Check sheet for the modelled part. Datum: model origin and axes. Units: mm. Coordinates: 2 decimals unless noted, no trailing zeros. Loops run counter-clockwise (first coordinate to the right, second up) from the corner with the lowest first, then second, coordinate; pieces in that order, holes last. Notation, with made-up numbers: (22, -39.75) -> (29, -39.75) arc R23 cw to (29, -5.75) -> close; hole circle Ø1 at (63.5, 17). An arc over 180 degrees is marked (long way). Use CSV: the item, a comma, the result in double quotes.
```python
from build123d import *

# Parameters (mm, degrees)
BOSS_EXTRUDE1_DEPTH = 60


with BuildPart() as part:
    # Sketch1 → Boss-Extrude1 (new body)
    with BuildSketch(Plane.XY.offset(12.5)):
        with BuildLine():
            Line((1.189339828, 2), (-1.189339828, 2))
            ThreePointArc((-1.189339828, 2), (-1.285010686, 2.019030117), (-1.366116524, 2.073223305))
            Line((-1.366116524, 2.073223305), (-3.116116524, 3.823223305))
            ThreePointArc((-3.116116524, 3.823223305), (-3.189339828, 4), (-3.116116524, 4.176776695))
            Line((-3.116116524, 4.176776695), (-2.292893219, 5))
            Line((-2.292893219, 5), (-3.094974747, 5))
            Line((-3.094974747, 5), (-3.623223305, 4.471751442))
            ThreePointArc((-3.623223305, 4.471751442), (-3.8, 4.398528137), (-3.976776695, 4.471751442))
            Line((-3.976776695, 4.471751442), (-4.505025253, 5))
            Line((-4.505025253, 5), (-4.75, 5))
            ThreePointArc((-4.75, 5), (-4.926776695, 4.926776695), (-5, 4.75))
            Line((-5, 4.75), (-5, 4.505025253))
            Line((-5, 4.505025253), (-4.471751442, 3.976776695))
            ThreePointArc((-4.471751442, 3.976776695), (-4.398528137, 3.8), (-4.471751442, 3.623223305))
            Line((-4.471751442, 3.623223305), (-5, 3.094974747))
            Line((-5, 3.094974747), (-5, 2.292893219))
            Line((-5, 2.292893219), (-4.176776695, 3.116116524))
            ThreePointArc((-4.176776695, 3.116116524), (-4, 3.189339828), (-3.823223305, 3.116116524))
            Line((-3.823223305, 3.116116524), (-2.073223305, 1.366116524))
            ThreePointArc((-2.073223305, 1.366116524), (-2.019030117, 1.285010686), (-2, 1.189339828))
            Line((-2, 1.189339828), (-2, -1.189339828))
            ThreePointArc((-2, -1.189339828), (-2.019030117, -1.285010686), (-2.073223305, -1.366116524))
            Line((-2.073223305, -1.366116524), (-3.823223305, -3.116116524))
            ThreePointArc((-3.823223305, -3.116116524), (-4, -3.189339828), (-4.176776695, -3.116116524))
            Line((-4.176776695, -3.116116524), (-5, -2.292893219))
            Line((-5, -2.292893219), (-5, -3.094974747))
            Line((-5, -3.094974747), (-4.471751442, -3.623223305))
            ThreePointArc((-4.471751442, -3.623223305), (-4.398528137, -3.8), (-4.471751442, -3.976776695))
            Line((-4.471751442, -3.976776695), (-5, -4.505025253))
            Line((-5, -4.505025253), (-5, -4.75))
            ThreePointArc((-5, -4.75), (-4.926776695, -4.926776695), (-4.75, -5))
            Line((-4.75, -5), (-4.505025253, -5))
            Line((-4.505025253, -5), (-3.976776695, -4.471751442))
            ThreePointArc((-3.976776695, -4.471751442), (-3.8, -4.398528137), (-3.623223305, -4.471751442))
            Line((-3.623223305, -4.471751442), (-3.094974747, -5))
            Line((-3.094974747, -5), (-2.292893219, -5))
            Line((-2.292893219, -5), (-3.116116524, -4.176776695))
            ThreePointArc((-3.116116524, -4.176776695), (-3.189339828, -4), (-3.116116524, -3.823223305))
            Line((-3.116116524, -3.823223305), (-1.366116524, -2.073223305))
            ThreePointArc((-1.366116524, -2.073223305), (-1.285010686, -2.019030117), (-1.189339828, -2))
            Line((-1.189339828, -2), (1.189339828, -2))
            ThreePointArc((1.189339828, -2), (1.285010686, -2.019030117), (1.366116524, -2.073223305))
            Line((1.366116524, -2.073223305), (3.116116524, -3.823223305))
            ThreePointArc((3.116116524, -3.823223305), (3.189339828, -4), (3.116116524, -4.176776695))
            Line((3.116116524, -4.176776695), (2.292893219, -5))
            Line((2.292893219, -5), (3.094974747, -5))
            Line((3.094974747, -5), (3.623223305, -4.471751442))
            ThreePointArc((3.623223305, -4.471751442), (3.8, -4.398528137), (3.976776695, -4.471751442))
            Line((3.976776695, -4.471751442), (4.505025253, -5))
            Line((4.505025253, -5), (4.75, -5))
            ThreePointArc((4.75, -5), (4.926776695, -4.926776695), (5, -4.75))
            Line((5, -4.75), (5, -4.505025253))
            Line((5, -4.505025253), (4.471751442, -3.976776695))
            ThreePointArc((4.471751442, -3.976776695), (4.398528137, -3.8), (4.471751442, -3.623223305))
            Line((4.471751442, -3.623223305), (5, -3.094974747))
            Line((5, -3.094974747), (5, -2.292893219))
            Line((5, -2.292893219), (4.176776695, -3.116116524))
            ThreePointArc((4.176776695, -3.116116524), (4, -3.189339828), (3.823223305, -3.116116524))
            Line((3.823223305, -3.116116524), (2.073223305, -1.366116524))
            ThreePointArc((2.073223305, -1.366116524), (2.019030117, -1.285010686), (2, -1.189339828))
            Line((2, -1.189339828), (2, 1.189339828))
            ThreePointArc((2, 1.189339828), (2.019030117, 1.285010686), (2.073223305, 1.366116524))
            Line((2.073223305, 1.366116524), (3.823223305, 3.116116524))
            ThreePointArc((3.823223305, 3.116116524), (4, 3.189339828), (4.176776695, 3.116116524))
            Line((4.176776695, 3.116116524), (5, 2.292893219))
            Line((5, 2.292893219), (5, 3.094974747))
            Line((5, 3.094974747), (4.471751442, 3.623223305))
            ThreePointArc((4.471751442, 3.623223305), (4.398528137, 3.8), (4.471751442, 3.976776695))
            Line((4.471751442, 3.976776695), (5, 4.505025253))
            Line((5, 4.505025253), (5, 4.75))
            ThreePointArc((5, 4.75), (4.926776695, 4.926776695), (4.75, 5))
            Line((4.75, 5), (4.505025253, 5))
            Line((4.505025253, 5), (3.976776695, 4.471751442))
            ThreePointArc((3.976776695, 4.471751442), (3.8, 4.398528137), (3.623223305, 4.471751442))
            Line((3.623223305, 4.471751442), (3.094974747, 5))
            Line((3.094974747, 5), (2.292893219, 5))
            Line((2.292893219, 5), (3.116116524, 4.176776695))
            ThreePointArc((3.116116524, 4.176776695), (3.189339828, 4), (3.116116524, 3.823223305))
            Line((3.116116524, 3.823223305), (1.366116524, 2.073223305))
            ThreePointArc((1.366116524, 2.073223305), (1.285010686, 2.019030117), (1.189339828, 2))
        make_face()
    extrude(amount=-BOSS_EXTRUDE1_DEPTH)


solid = part.part
```
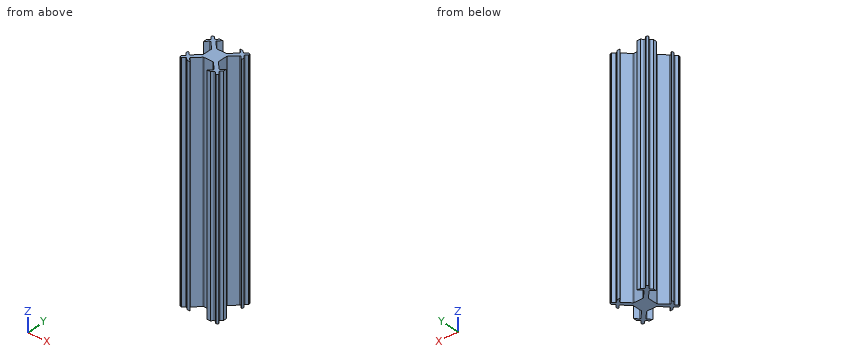
1) Go/stop test with flat-tipped pins: pin 1 Ø1.9 at (y, z) = (0.5, -6) entering from -X; pin 2 Ø2.5 at (y, z) = (0, -22) entering from +X; pin 3 Ø3 at (x, y) = (-4, 0.5) entering from +Z; pin 4 Ø1.9 at (x, z) = (-0.5, -25) entering from +Y. Record where each tip stops, or that it passes through.
Answer below:
pin 1,"stops at x = -2.16"
pin 2,"stops at x = 2.01"
pin 3,"passes through"
pin 4,"stops at y = 2.16"
2) Thickness scan on line 1 along X through (y, z) = (4, 6); line 2 along Y through (x, z) = (2.5, -21); line 3 along Y through (x, z) = (-3, -44). Record the ranges inside material, lowest first. Write a range as from..to.
Answer below:
line 1,"x = -4.49..-3.19, 3.19..4.49"
line 2,"y = -5..-4.79, -3.21..-1.79, 1.79..3.21, 4.79..5"
line 3,"y = -5..-4.29, -3.71..-2.29, 2.29..3.71, 4.29..5"
3) Cross-section at A-A on y = 0.5. Record the boundary of the cut face in (x, z).
Answer below:
outline,"(-2, -47.5) -> (2, -47.5) -> (2, 12.5) -> (-2, 12.5) -> close"
